Part model, mm, in its own coordinate system. Face numbers are marked on the shaded views. A direction names the side the tool comes from. Coordinates: 2 decimals unless noted, no trailing zeros. Loops run counter-clockwise (first coordinate to the right, second up) from the corner with the lowest first, then second, coordinate; pieces in that order, holes last. Notation, with made-up numbers: (45, -10) - (93, -10) arc R18 cw to (93, 21) - close; hole circle Ø2 at (33.5, 5.5). An arc over 180 degrees is marked (long way). Use a Markdown table: item, result. Add a question column.
1) Pull direction Y, two halves, no side cores. Call the marked faces 3 and 4: +Y half, -Y half, draft (parallel to the pull), parting line (faces both ways), or undercut.
2) Drop flat-ended pins along their axis: P1, Ø3, axis at y = 28, z = -3.5, coming from the +X side; P2, Ø3, axis at y = 17.5, z = 1.5, coming from the +X side; P3, Ø10, axis at x = 36.5, z = 14, coming from the +Y side. Give the stop position or say it passes through.
3) Band-saw the part on B-B (y = 0). Give the cut face in (x, z) (3 decimals).
4) Tool access for the marked faces 1 and 2: list every direction of +Z, -Z, +X, -X, +Y, -Y with a clear straight run to the whole face (end or side of a thin tool).
5) Probe probe 1 along Y at (x, z) = (43, 0) (3 decimals); probe 2 along Y at (x, z) = (33.5, 18) (3 decimals). List the from-to ranges inside material, lowest first. Write a range as [from, to].
6) Band-saw the part on C-C (x = 52). Give the cut face in (y, z) (3 decimals).
7) Band-saw the part on A-A (z = 0). Give the cut face in (x, y) (3 decimals).
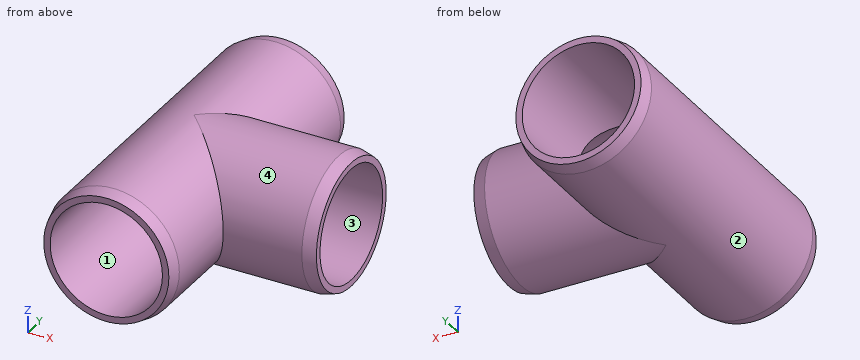
from build123d import *

# Parameters (mm, degrees)
F0_R          = 24.765
F0_R_2        = 21.082
F1_DEPTH      = 59.055
F2_R          = 24.765
F2_R_2        = 21.082
F3_DEPTH      = 59.055
F4_DEPTH      = 59.0560001
F5_DEPTH      = 59.0560001
F5_DEPTH_BACK = 59.0560001
F6_SIZE2      = 1.27
F6_SIZE       = 4.7397045256
F6_2_SIZE2    = 1.27
F6_2_SIZE     = 4.7397045256


# Not quite as in the source:
# - two fillets or chamfers of one size are made in one step


with BuildPart() as f1:
    # F0 (on Front) → F1 (new body, symmetric)
    with BuildSketch(Plane.XZ):
        Circle(F0_R)
        Circle(F0_R_2, mode=Mode.SUBTRACT)
    extrude(amount=F1_DEPTH, both=True)

    # F2 (on Right) → F3 (join)
    with BuildSketch(Plane.YZ):
        Circle(F2_R)
        Circle(F2_R_2, mode=Mode.SUBTRACT)
    extrude(amount=F3_DEPTH)

    # F2 (on Right) → F4 (cut, through all)
    with BuildSketch(Plane.YZ):
        Circle(F2_R_2)
    extrude(amount=F4_DEPTH, mode=Mode.SUBTRACT)

    # F0 (on Front) → F5 (cut, two sides)
    with BuildSketch(Plane.XZ) as f5_sk:
        Circle(F0_R_2)
    extrude(amount=F5_DEPTH, mode=Mode.SUBTRACT)
    extrude(f5_sk.sketch, amount=-F5_DEPTH_BACK, mode=Mode.SUBTRACT)

    # F6
    f6_edges = [f1.edges().sort_by_distance(p)[0] for p in [
        (-24.765, -59.055, 0),
        (-24.765, 59.055, 0),
    ]]
    f6_side = f1.faces().sort_by_distance((-24.765, 0, 0))[0]
    chamfer(f6_edges, length=F6_SIZE, length2=F6_SIZE2, reference=f6_side)

    # F6#2
    f6_2_edges = [f1.edges().sort_by_distance(p)[0] for p in [
        (59.055, -24.765, 0),
    ]]
    f6_2_side = f1.faces().sort_by_distance((29.5275, -24.765, 0))[0]
    chamfer(f6_2_edges, length=F6_2_SIZE, length2=F6_2_SIZE2, reference=f6_2_side)


solid = f1.part
Answer block:
| question | item | result |
|---|---|---|
| 1 | face 3 | undercut |
| 1 | face 4 | parting line |
| 2 | P1 | x = 24.68 |
| 2 | P2 | x = -20.87 |
| 2 | P3 | y = 23.07 |
| 3 | outline | (0, -24.765) - (54.315, -24.765) - (59.055, -23.495) - (59.055, -21.082) - (0, -21.082) arc R21.082 cw to (0, 21.082) - (59.055, 21.082) - (59.055, 23.495) - (54.315, 24.765) - (0, 24.765) arc R24.765 ccw to start |
| 4 | face 1 | +Y, -Y |
| 4 | face 2 | none |
| 5 | probe 1 | [-24.765, -21.082], [21.082, 24.765] |
| 5 | probe 2 | [-17.009, -10.975], [10.975, 17.009] |
| 6 | outline | circle Ø49.53 at (0, 0); hole circle Ø42.164 at (0, 0) |
| 7 | outline | (-24.765, -54.315) - (-23.495, -59.055) - (-21.082, -59.055) - (-21.082, 59.055) - (-23.495, 59.055) - (-24.765, 54.315) - close; (21.082, -59.055) - (23.495, -59.055) - (24.765, -54.315) - (24.765, -24.765) - (54.315, -24.765) - (59.055, -23.495) - (59.055, -21.082) - (21.082, -21.082) - close; (21.082, 21.082) - (59.055, 21.082) - (59.055, 23.495) - (54.315, 24.765) - (24.765, 24.765) - (24.765, 54.315) - (23.495, 59.055) - (21.082, 59.055) - close |
